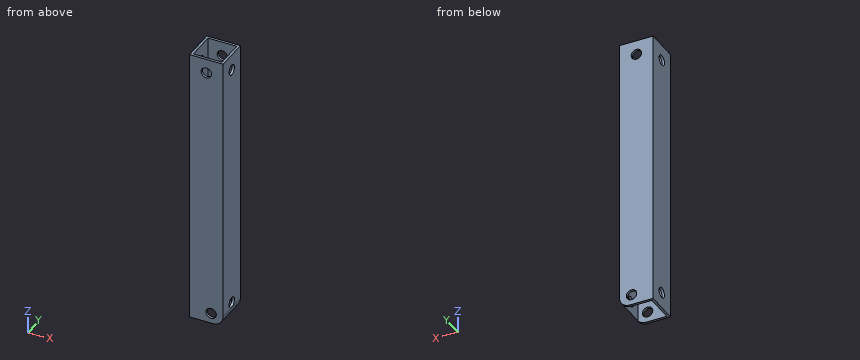
from build123d import *

# Parameters (mm, degrees)
CROQUIS1_W              = 42
CROQUIS1_H              = 42
SALIENTE_EXTRUIR1_DEPTH = 175
CORTAR_EXTRUIR1_DEPTH   = 355.297078735
CROQUIS3_R              = 6.5
CORTAR_EXTRUIR3_DEPTH   = 60
CROQUIS4_R              = 6.5
CORTAR_EXTRUIR4_DEPTH   = 70
CROQUIS5_R              = 6.5
CORTAR_EXTRUIR5_DEPTH   = 182.190507478
REDONDEO1_R             = 13
CROQUIS6_R              = 6.5
CORTAR_EXTRUIR6_DEPTH   = 60


with BuildPart() as part:
    # Croquis1 → Saliente-Extruir1 (new, symmetric)
    with BuildSketch(Plane.XY):
        Rectangle(CROQUIS1_W, CROQUIS1_H)
    extrude(amount=SALIENTE_EXTRUIR1_DEPTH, both=True)

    # Croquis3D1 → Cortar-Extruir1 (cut, through all)
    with BuildSketch(Plane(origin=(-17.9, -17.9, 175), x_dir=(0.7071067811865475, 0.7071067811865477, 0), z_dir=(0, 0, 1))):
        Polygon((0, 0), (25.314422766, -25.314422766), (50.628845533, 0), (25.314422766, 25.314422766), align=None)
    extrude(amount=-CORTAR_EXTRUIR1_DEPTH, mode=Mode.SUBTRACT)

    # Croquis3 → Cortar-Extruir3 (cut)
    with BuildSketch(Plane.XZ.offset(21)):
        with Locations((0, 157)):
            Circle(CROQUIS3_R)
    extrude(amount=-CORTAR_EXTRUIR3_DEPTH, mode=Mode.SUBTRACT)

    # Croquis4 → Cortar-Extruir4 (cut)
    with BuildSketch(Plane(origin=(21, 0, 0), x_dir=(0, 0, -1), z_dir=(1, 0, 0))):
        with Locations(Location((155, 0, 0), (0, 0, 90))):
            Circle(CROQUIS4_R)
    extrude(amount=-CORTAR_EXTRUIR4_DEPTH, mode=Mode.SUBTRACT)

    # Croquis5 → Cortar-Extruir5 (cut, through all)
    with BuildSketch(Plane(origin=(0, 21, 0), x_dir=(1, 0, 0), z_dir=(0, 1, 0))):
        with Locations(Location((6, 162, 0), (0, 0, 180))):
            Circle(CROQUIS5_R)
    extrude(amount=-CORTAR_EXTRUIR5_DEPTH, mode=Mode.SUBTRACT)

    # Redondeo1
    # the kernel refuses this fillet: 13 mm, written as the material it takes off along each edge
    with BuildSketch(Plane(origin=(21, 53.5, -175), x_dir=(0, 0, 1), z_dir=(0, -1, 0))) as redondeo1_piece_1:
        with BuildLine():
            CenterArc((REDONDEO1_R, REDONDEO1_R), REDONDEO1_R, 180, 90)
            Line((0, REDONDEO1_R), (0, 0))
            Line((0, 0), (REDONDEO1_R, 0))
        make_face()
    extrude(amount=107, mode=Mode.SUBTRACT)

    # Croquis6 → Cortar-Extruir6 (cut)
    with BuildSketch(Plane.ZY.offset(21)):
        with Locations(Location((155, 0, 0), (0, 0, 270))):
            Circle(CROQUIS6_R)
    extrude(amount=-CORTAR_EXTRUIR6_DEPTH, mode=Mode.SUBTRACT)


solid = part.part
The listing builds one solid part. Answer for the finished solid, in the listing's coordinates (mm). Coordinates: 2 decimals unless noted, no trailing zeros. Write each loop counter-clockwise with the first axis right and the second up, starting at its lowest first coordinate (ties: lowest second). Pieces come first, ordered by that corner, then holes. Notation, with made-up numbers: (77, 38) - (111, 38) arc R8 ccw to (111, 46) - close; hole circle Ø8 at (43, 72.25). An arc over 180 degrees is marked (long way). Return JSON: item names as keys, results as strings.
1. The part is cut by section A-A on z = 20.5. Determine the outline of the cut face in (x, y), then the cut area to 3 significant figures.
Final values:
{"outline": "(-21, -21) - (21, -21) - (21, 21) - (-21, 21) - close; hole (-17.9, -17.9) - (17.9, -17.9) - (17.9, 17.9) - (-17.9, 17.9) - close", "area": "482 mm^2"}
2. This flat-tipped pin is pushed along its axis until it touches: pin 1 Ø11.5 at (x, z) = (6, -162) entering from +Y. Where does it stop, or does it pass through?
Final values:
{"pin 1": "through"}
3. Consider line 1 along Z through (x, y) = (-18.9, 0); line 2 along X through (y, z) = (-16, -37). Determine where each line is inside the solid, lowest interval first.
Final values:
{"line 1": "-175 to -161.5, -148.5 to 148.5, 161.5 to 175", "line 2": "-21 to -17.9, 17.9 to 21"}
4. The part is cut by section C-C on x = 3. Determine the outline of the cut face in (y, z), then the cut area to 3 significant figures.
Final values:
{"outline": "(-21, -175) - (-17.9, -175) - (-17.9, -167.77) - (-21, -167.77) - close; (-21, -156.23) - (-17.9, -156.23) - (-17.9, 151.23) - (-21, 151.23) - close; (-21, 162.77) - (-17.9, 162.77) - (-17.9, 175) - (-21, 175) - close; (17.9, -175) - (21, -175) - (21, -167.77) - (17.9, -167.77) - close; (17.9, -156.23) - (21, -156.23) - (21, 151.23) - (17.9, 151.23) - close; (17.9, 162.77) - (21, 162.77) - (21, 175) - (17.9, 175) - close", "area": "2,030 mm^2"}
5. The part is cut by section B-B on y = 13.5. Determine the outline of the cut face in (x, z), then the cut area to 3 significant figures.
Final values:
{"outline": "(-21, -175) - (-17.9, -175) - (-17.9, 175) - (-21, 175) - close; (17.9, -170.43) arc R13 ccw to (21, -162) - (21, 175) - (17.9, 175) - close", "area": "2,150 mm^2"}
